```python
from build123d import *

# Parameters (mm, degrees)
SKETCH1_W           = 75
SKETCH1_H           = 42.05
SKETCH1_R           = 2
BOSS_EXTRUDE2_DEPTH = 4.25


with BuildPart() as part:
    # Sketch1 → Boss-Extrude2 (new body)
    with BuildSketch(Plane.XY):
        with Locations((-2.5, -11.725)):
            Rectangle(SKETCH1_W, SKETCH1_H)
        with Locations((-25, 0)):
            Circle(SKETCH1_R, mode=Mode.SUBTRACT)
        with Locations((25, 0)):
            Circle(SKETCH1_R, mode=Mode.SUBTRACT)
        with BuildLine():
            ThreePointArc((-8.09596287, -19.913215449), (0, -29.75), (8.09596287, -19.913215449))
            Line((8.09596287, -19.913215449), (6.3, -10.75))
            Line((6.3, -10.75), (6.3, 0))
            ThreePointArc((6.3, 0), (0, 6.3), (-6.3, 0))
            Line((-6.3, 0), (-6.3, -10.75))
            Line((-6.3, -10.75), (-8.09596287, -19.913215449))
        make_face(mode=Mode.SUBTRACT)
    extrude(amount=BOSS_EXTRUDE2_DEPTH)


solid = part.part
```
Source: CAD feature listing. Evaluate the final solid. Frame: model axes, mm. A direction names the side the tool comes from. Round coordinates to 2 decimals unless told otherwise and drop trailing zeros. Loops run counter-clockwise (first coordinate to the right, second up) from the corner with the lowest first, then second, coordinate; pieces in that order, holes last.
1. Mould query, pull axis X, two halves, no side actions, for faces 1 (the flat face through (-3, 9.3, 2)), 2 (the flat face through (6.3, -5, 2)), 3 (the flat face through (-40, -12, 2)). Classes: released by +X, released by -X, zero draft, split by the parting line, or undercut.
2. Section query C-C on x = 25. Output: boundary loops of the cut face in (y, z), and give its area (3 significant figures).
3. Access query for faces 4 (the flat face through (-7.185, -15.267, 2.095)), 5 (the flat face through (-11, -11, 4.25)). Directions: +Z, -Z, +X, -X, +Y, -Y. A direction counts if a zero-diameter tool reaches every point of the face in a straight line with its end or side. Return the directions, or none.
4. Ray query, L1, parallel to X at y = -3.5, z = 1.2; L2, parallel to X at y = -21.5, z = 2.85; L3, parallel to Y at x = 25, z = 1.1. Return the intervals inside material, ascending.
5. Section query A-A on y = -21.5. Output: boundary loops of the cut face in (x, z), and give its area (3 significant figures).
6. Contact query for a flat-ended pin moving along its axis: pin 1 (2.5 mm diameter, centred on x = -25, y = 0, fed in from -Z). Output: stop coordinate, or through.
7. Section query B-B on z = 1.7. Output: boundary loops of the cut face in (x, y), and give its area (3 significant figures).
Answers below:
1. face 1: zero draft
1. face 2: undercut
1. face 3: released by -X
2. outline: (-32.75, 0) - (-2, 0) - (-2, 4.25) - (-32.75, 4.25) - close; (2, 0) - (9.3, 0) - (9.3, 4.25) - (2, 4.25) - close
2. area: 162 mm2
3. face 4: +Z, -Z
3. face 5: +Z, +X, -X, +Y, -Y
4. L1: x = -40 to -6.3, 6.3 to 35
4. L2: x = -40 to -8.25, 8.25 to 35
4. L3: y = -32.75 to -2, 2 to 9.3
5. outline: (-40, 0) - (-8.25, 0) - (-8.25, 4.25) - (-40, 4.25) - close; (8.25, 0) - (35, 0) - (35, 4.25) - (8.25, 4.25) - close
5. area: 249 mm2
6. pin 1: passes through
7. outline: (-40, -32.75) - (35, -32.75) - (35, 9.3) - (-40, 9.3) - close; hole circle Ø4 at (-25, 0); hole (-8.1, -19.91) arc R8.25 ccw (long way) to (8.1, -19.91) - (6.3, -10.75) - (6.3, 0) arc R6.3 ccw to (-6.3, 0) - (-6.3, -10.75) - close; hole circle Ø4 at (25, 0)
7. area: 2,670 mm2
